from build123d import *

# Parameters (mm, degrees)
F0_W          = 50.8
F0_H          = 50.8
F1_DEPTH      = 381
F2_R          = 11.1125
F3_DEPTH      = 215.9
F5_DEPTH      = 4.7625
F5_DEPTH_BACK = 4.7625


# Not quite as in the source:
# - the program builds the solid bodies; features that only make, move or delete a surface that nothing else refers to are left out


with BuildPart() as f1:
    # F0 (on Top) → F1 (new body)
    with BuildSketch(Plane.XY):
        Rectangle(F0_W, F0_H)
    extrude(amount=F1_DEPTH)

    # F2 (on face) → F3 (join)
    with BuildSketch(Plane.XZ.offset(25.4)):
        with Locations((0, 341.3125)):
            Circle(F2_R)
    extrude(amount=F3_DEPTH)

    # F4 (on Right) → F5 (join, two sides)
    with BuildSketch(Plane.YZ) as f5_sk:
        Polygon((-292.1, 330.2), (-241.3, 330.2), (-241.3, 365.125), (-247.65, 365.125), (-292.1, 336.55), align=None)
    extrude(amount=F5_DEPTH)
    extrude(f5_sk.sketch, amount=-F5_DEPTH_BACK)


solid = f1.part
Work out the finished part from the listing and answer in its coordinate system (mm). A direction names the side the tool comes from. Give positions to 0.01 mm unless a question says otherwise; leave off trailing zeros. Loops run counter-clockwise (first coordinate to the right, second up) from the corner with the lowest first, then second, coordinate; pieces in that order, holes last. Notation, with made-up numbers: (63.5, 20.5) -> (87.5, 20.5) arc R19 cw to (87.5, 38.5) -> close; hole circle Ø3 at (-1, -27). An arc over 180 degrees is marked (long way). Use a Markdown table: item, result. Add a question column.
1) The part is cut by section B-B, the plane z = 199.5. Determine the outline of the cut face in (x, y), plus the area to 3 significant figures.
2) Which of the six approach directions +Z, -Z, +X, -X, +Y, -Y give full straight-line access (tool end or side, diameter ignored) to faces 1 (the flat face through (4.762, -261, 344)), 2 (the flat face through (0, 25.4, 188)), 3 (the flat face through (0, -267, 330.2)), 4 (the flat face through (-4.762, -261, 344)), 5 (the cylindrical face through (-8.82, -131.84, 334.55))?
3) The part is cut by section A-A, the plane x = 18. Determine the outline of the cut face in (y, z).
4) The part is cut by section C-C, the plane y = -220. Determine the outline of the cut face in (x, z) (1 decimal), plus the area to 3 significant figures.
5) Consider line 1 along Y through (x, z) = (-8, 350.5); line 2 along Z through (x, y) = (5.5, -53.5); line 3 along Z through (x, y) = (-8, -92.5). Determine where each line is inside the solid, lowest interval first.
6) Each of these flat-tipped pins is pushed along its axis until it touches: P1, Ø1.5, axis at x = 5.5, y = -64, coming from the +Z side; P2, Ø3, axis at x = -9, z = 340, coming from the -Y side; P3, Ø8, axis at x = 9.5, y = -71, coming from the -Z side. Where does it stop, or does it pass through?
Reported:
| question | item | result |
|---|---|---|
| 1 | outline | (-25.4, -25.4) -> (25.4, -25.4) -> (25.4, 25.4) -> (-25.4, 25.4) -> close |
| 1 | area | 2,580 mm^2 |
| 2 | face 1 | +Z, -Z, +X, -Y |
| 2 | face 2 | +Z, -Z, +X, -X, +Y |
| 2 | face 3 | -Z, +X, -X, -Y |
| 2 | face 4 | +Z, -Z, -X, -Y |
| 2 | face 5 | none |
| 3 | outline | (-25.4, 0) -> (25.4, 0) -> (25.4, 381) -> (-25.4, 381) -> close |
| 4 | outline | circle Ø22.2 at (0, 341.3) |
| 4 | area | 388 mm^2 |
| 5 | line 1 | y = -25.4 to 25.4 |
| 5 | line 2 | z = 331.66 to 350.97 |
| 5 | line 3 | z = 333.6 to 349.03 |
| 6 | P1 | stops at z = 351.36 |
| 6 | P2 | stops at y = -241.3 |
| 6 | P3 | stops at z = 331.66 |
